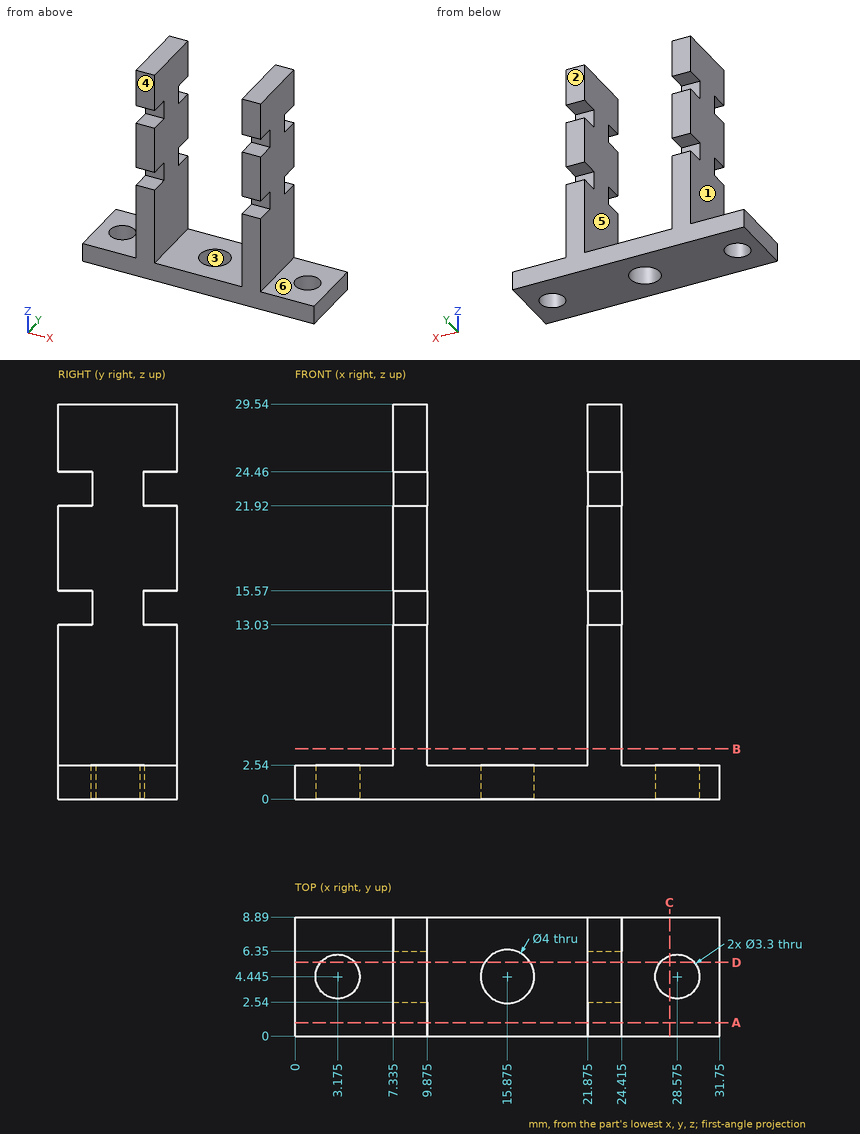
Answer from the drawing. Dimensions are ordinates in mm from the lowest x, y and z of the part. A direction names the side the tool comes from. Give positions to 0.01 mm unless a question says otherwise; leave off trailing zeros. Loops run counter-clockwise (first coordinate to the right, second up) from the corner with the lowest first, then second, coordinate; pieces in that order, holes last. Notation, with made-up numbers: (-28, 72) -> (25, 72) arc R9 ccw to (25, 87) -> close; hole circle Ø9 at (-5.5, -20.5). An arc over 180 degrees is marked (long way). Answer as CSV lines item,"result".
Item 1: Each of these flat-tipped pins is pushed along its axis until it touches: pin 1 (2.5 mm diameter, centred on x = 13.5, y = 4.5, fed in from +Z); pin 2 (4.5 mm diameter, centred on y = 2.5, z = 12.5, fed in from +X) (3 decimals); pin 3 (1.3 mm diameter, centred on x = 23.5, z = 14.5, fed in from +Y). Where does it stop, or does it pass through?
Returned:
pin 1,"stops at z = 2.54"
pin 2,"stops at x = 24.415"
pin 3,"stops at y = 6.35"
Item 2: For the marked faces 4, 5 and 6, determine the directions among +Z, -Z, +X, -X, +Y, -Y from which every point of the face is accessible in a straight line to the end or side of a thin tool.
Returned:
face 4,"+Z, -Z, +X, -X, -Y"
face 5,"+Z, +Y, -Y"
face 6,"+Z, +X, +Y, -Y"
Item 3: Consider line 1 (Z direction, x = 23.5, y = 6.75); line 2 (X direction, y = 0.75, z = 4.75) (3 decimals); line 3 (Z direction, x = 24.5, y = 2.5). Determine where each line is inside the solid, lowest interval first. Write a range as [from, to].
Returned:
line 1,"z = [0, 13.03], [15.57, 21.92], [24.46, 29.54]"
line 2,"x = [7.335, 9.875], [21.875, 24.415]"
line 3,"z = [0, 2.54]"
Item 4: Find section B-B on z = 3.75. Give the vertices of the cut face in (x, y) (3 decimals), plus the area to 3 significant figures.
Returned:
outline,"(7.335, 0) -> (9.875, 0) -> (9.875, 8.89) -> (7.335, 8.89) -> close; (21.875, 0) -> (24.415, 0) -> (24.415, 8.89) -> (21.875, 8.89) -> close"
area,"45.2 mm²"
Item 5: Find section C-C on x = 28. Give the vertices of the cut face in (y, z), plus the area to 3 significant figures.
Returned:
outline,"(0, 0) -> (2.9, 0) -> (2.9, 2.54) -> (0, 2.54) -> close; (5.99, 0) -> (8.89, 0) -> (8.89, 2.54) -> (5.99, 2.54) -> close"
area,"14.7 mm²"
Item 6: Determine the mould class of the marked faces 1, 2 and 3 for opening direction X: +X half, -X half, draft (parallel to the pull), parting line (faces both ways), or undercut.
Returned:
face 1,"-X half"
face 2,"draft"
face 3,"undercut"
Item 7: Find section D-D on y = 5.5. Give the vertices of the cut face in (x, z) (3 decimals).
Returned:
outline,"(0, 0) -> (1.906, 0) -> (1.906, 2.54) -> (0, 2.54) -> close; (4.444, 0) -> (14.176, 0) -> (14.176, 2.54) -> (9.875, 2.54) -> (9.875, 29.54) -> (7.335, 29.54) -> (7.335, 2.54) -> (4.444, 2.54) -> close; (17.574, 0) -> (27.306, 0) -> (27.306, 2.54) -> (24.415, 2.54) -> (24.415, 29.54) -> (21.875, 29.54) -> (21.875, 2.54) -> (17.574, 2.54) -> close; (29.844, 0) -> (31.75, 0) -> (31.75, 2.54) -> (29.844, 2.54) -> close"
Item 8: Find section A-A on y = 1. Give the vertices of the cut face in (x, z) (3 decimals), plus the area to 3 significant figures.
Returned:
outline,"(0, 0) -> (31.75, 0) -> (31.75, 2.54) -> (24.415, 2.54) -> (24.415, 13.03) -> (21.875, 13.03) -> (21.875, 2.54) -> (9.875, 2.54) -> (9.875, 13.03) -> (7.335, 13.03) -> (7.335, 2.54) -> (0, 2.54) -> close; (7.335, 15.57) -> (9.875, 15.57) -> (9.875, 21.92) -> (7.335, 21.92) -> close; (7.335, 24.46) -> (9.875, 24.46) -> (9.875, 29.54) -> (7.335, 29.54) -> close; (21.875, 15.57) -> (24.415, 15.57) -> (24.415, 21.92) -> (21.875, 21.92) -> close; (21.875, 24.46) -> (24.415, 24.46) -> (24.415, 29.54) -> (21.875, 29.54) -> close"
area,"192 mm²"
